from build123d import *

# Parameters (mm, degrees)
CROQUIS1_R              = 4.85
SALIENTE_EXTRUIR1_DEPTH = 3


with BuildPart() as part:
    # Croquis1 → Saliente-Extruir1 (new body)
    with BuildSketch(Plane(origin=(0, 0, 0), x_dir=(1, 0, 0), z_dir=(0, 1, 0))):
        Polygon((3, 10), (3, 0), (10, 0), (10, 3), (20, 3), (20, 0), (25, 0), (30, 0), (30, 3), (40, 3), (40, 0), (47, 0), (47, 10), (50, 10), (50, 20), (47, 20), (47, 30), (50, 30), (50, 40), (47, 40), (47, 50), (3, 50), (3, 40), (0, 40), (0, 30), (3, 30), (3, 20), (0, 20), (0, 10), align=None)
        with Locations(Location((25, 33, 0), (0, 0, 270))):
            Circle(CROQUIS1_R, mode=Mode.SUBTRACT)
    extrude(amount=SALIENTE_EXTRUIR1_DEPTH)


solid = part.part
For this review, take the finished solid that the model builds, in its own axes (mm). A direction names the side the tool comes from. Round coordinates to 2 decimals unless told otherwise and drop trailing zeros. Write each loop counter-clockwise with the first axis right and the second up, starting at its lowest first coordinate (ties: lowest second). Pieces come first, ordered by that corner, then holes. Notation, with made-up numbers: (62.5, 21.5) - (79.5, 21.5) arc R24 cw to (79.5, 39.5) - close; hole circle Ø7 at (-9, 40.5). An arc over 180 degrees is marked (long way). Use a Markdown table: item, result.
Q1. Wall thickness on line 1 along X through (y, z) = (2.3, -33); line 2 along X through (y, z) = (2.8, -22); line 3 along Z through (x, y) = (29, 0.6): over which ranges is each line inside the solid? List them lowest first.
Derived:
| item | result |
|---|---|
| line 1 | x = 0 to 20.15, 29.85 to 50 |
| line 2 | x = 3 to 47 |
| line 3 | z = -50 to -35.74, -30.26 to 0 |
Q2. We need section A-A (z = -33). Give the boundary of the cut face in (x, y).
Derived:
| item | result |
|---|---|
| outline | (0, 0) - (20.15, 0) - (20.15, 3) - (0, 3) - close; (29.85, 0) - (50, 0) - (50, 3) - (29.85, 3) - close |
Q3. Machinability: for faces 4 (the flat face through (47, 1, -25)), 5 (the flat face through (47, 1, -45)), 6 (the flat face through (20, 1, -2)), which of the approach directions +Z, -Z, +X, -X, +Y, -Y give a long, thin tool a straight path to every point of the face, cutting with its end or side? Answer none if there is none.
Derived:
| item | result |
|---|---|
| face 4 | +X, +Y, -Y |
| face 5 | -Z, +X, +Y, -Y |
| face 6 | +Z, +Y, -Y |
Q4. We need section B-B (x = 25). Give the boundary of the cut face in (y, z), plus the area to 3 significant figures.
Derived:
| item | result |
|---|---|
| outline | (0, -50) - (3, -50) - (3, -37.85) - (0, -37.85) - close; (0, -28.15) - (3, -28.15) - (3, 0) - (0, 0) - close |
| area | 121 mm2 |
Q5. Clearance check with flat-ended pins moving along their axes: pin 1 (0.9 mm diameter, centred on x = 2, y = 1, fed in from +Z); pin 2 (0.9 mm diameter, centred on y = 1, z = -25, fed in from +X); pin 3 (1.5 mm diameter, centred on x = 2, y = 1.5, fed in from -Z). State where each tip first meets the part, or that it passes through.
Derived:
| item | result |
|---|---|
| pin 1 | stops at z = -10 |
| pin 2 | stops at x = 47 |
| pin 3 | stops at z = -40 |
Q6. We need section D-D (x = 14.5). Give the boundary of the cut face in (y, z), plus the area to 3 significant figures.
Derived:
| item | result |
|---|---|
| outline | (0, -50) - (3, -50) - (3, -3) - (0, -3) - close |
| area | 141 mm2 |
Q7. The part is to be moulded in two halves that separate along Z. For faces 1 (the flat face through (48, 1, -10)), 2 (the flat face through (3, 1, -45)), 3 (the flat face through (1, 1, -30)), say which applies: pulls with the +Z half, pulls with the -Z half, needs draft (parallel to the pull), parting line crosses it, or undercut.
Derived:
| item | result |
|---|---|
| face 1 | pulls with the +Z half |
| face 2 | needs draft |
| face 3 | undercut |
